```python
from build123d import *

# Parameters (mm, degrees)
MAIN_PLATE_DEPTH                 = 3
TOP_PLATE_CONNECTOR_HOLES_DEPTH  = 37.224942593
ZIPTIE_STRUCTURE_DEPTH           = 6
SKETCH5_W                        = 7.5
SKETCH5_H                        = 3
ZIPTIE_HOLES_DEPTH               = 52.45154631
REMOVING_STRESS_CONCENTRATIONS_R = 1.5


with BuildPart() as part:
    # Sketch1 → Main Plate (new body)
    with BuildSketch(Plane(origin=(0, 0, 0), x_dir=(1, 0, 0), z_dir=(0, 1, 0))):
        Polygon((-7, 25.526911935), (7, 25.526911935), (25.526911935, 7), (25.526911935, -7), (7, -25.526911935), (-7, -25.526911935), (-25.526911935, -7), (-25.526911935, 7), align=None)
    extrude(amount=MAIN_PLATE_DEPTH)

    # Sketch2 → Top Plate Connector Holes (cut, through all)
    with BuildSketch(Plane.XZ):
        Polygon((10.960155108, 18.03122292), (18.03122292, 10.960155108), (15.909902577, 8.838834765), (8.838834765, 15.909902577), align=None)
        Polygon((8.838834765, -15.909902577), (15.909902577, -8.838834765), (18.03122292, -10.960155108), (10.960155108, -18.03122292), align=None)
        Polygon((-15.909902577, -8.838834765), (-8.838834765, -15.909902577), (-10.960155108, -18.03122292), (-18.03122292, -10.960155108), align=None)
        Polygon((-8.838834765, 15.909902577), (-15.909902577, 8.838834765), (-18.03122292, 10.960155108), (-10.960155108, 18.03122292), align=None)
    extrude(amount=-TOP_PLATE_CONNECTOR_HOLES_DEPTH, mode=Mode.SUBTRACT)

    # Sketch3 → ZipTie Structure (add)
    with BuildSketch(Plane.XZ):
        Polygon((1.767766953, 19.445436483), (19.445436483, 1.767766953), (17.324116139, -0.353553391), (-0.353553391, 17.324116139), align=None)
        Polygon((-1.767766953, -19.445436483), (0.353553391, -17.324116139), (-17.324116139, 0.353553391), (-19.445436483, -1.767766953), align=None)
    extrude(amount=ZIPTIE_STRUCTURE_DEPTH)

    # Sketch5 → ZipTie Holes (cut, through all)
    with BuildSketch(Plane(origin=(-10.606601718, 0, -10.606601718), x_dir=(-0.7071067811865475, 0, 0.7071067811865477), z_dir=(-0.7071067811865477, 0, -0.7071067811865475))):
        with Locations((-5.75, -1.5)):
            Rectangle(SKETCH5_W, SKETCH5_H)
        with Locations((5.75, -1.5)):
            Rectangle(SKETCH5_W, SKETCH5_H)
    extrude(amount=-ZIPTIE_HOLES_DEPTH, mode=Mode.SUBTRACT)

    # Removing Stress Concentrations
    removing_stress_concentrations_edges = [part.edges().sort_by_distance(p)[0] for p in [
        (8.131727984, -3, 10.960155108),
        (10.960155108, -3, 8.131727984),
        (16.263455967, -3, 2.828427125),
        (-2.828427125, -3, -16.263455967),
        (-8.131727984, -3, -10.960155108),
        (-10.960155108, -3, -8.131727984),
        (-16.263455967, -3, -2.828427125),
        (2.828427125, -3, 16.263455967),
        (-16.263455967, 0, -2.828427125),
        (-8.131727984, 0, -10.960155108),
        (-0.707106781, 0, -18.384776311),
        (2.828427125, 0, 18.384776311),
        (10.606601718, 0, 10.606601718),
        (18.384776311, 0, 2.828427125),
        (10.960155108, 0, 8.131727984),
        (2.828427125, 0, 16.263455967),
        (0.707106781, -6, 18.384776311),
        (18.384776311, -6, 0.707106781),
        (18.384776311, 0, 0.707106781),
        (16.263455967, 0, 2.828427125),
        (0.707106781, 0, 18.384776311),
        (8.131727984, 0, 10.960155108),
        (-18.384776311, 0, -0.707106781),
        (-2.828427125, 0, -16.263455967),
        (-10.960155108, 0, -8.131727984),
        (-2.828427125, 0, -18.384776311),
        (-10.606601718, 0, -10.606601718),
        (-18.384776311, 0, -2.828427125),
        (-18.384776311, -6, -0.707106781),
        (-0.707106781, -6, -18.384776311),
    ]]
    fillet(removing_stress_concentrations_edges, radius=REMOVING_STRESS_CONCENTRATIONS_R - 0.0001)  # a hair under: the kernel refuses the full size


solid = part.part
```
Here's how the part is built. I have some questions about the finished solid (model axes, mm). A direction names the side the tool comes from. Give positions to 0.01 mm unless a question says otherwise; leave off trailing zeros. Write each loop counter-clockwise with the first axis right and the second up, starting at its lowest first coordinate (ties: lowest second). Pieces come first, ordered by that corner, then holes.
(1) Imagine slicing it at A-A, the plane y = -3.75. Write out the boundary of the cut face in (x, z), and give its area (3 significant figures).
Output values:
outline: (-19.45, -1.77) - (-1.77, -19.45) - (0.35, -17.32) - (-17.32, 0.35) - close; (-0.35, 17.32) - (17.32, -0.35) - (19.45, 1.77) - (1.77, 19.45) - close
area: 150 mm2
(2) On a 3-axis mill with a long thin cutter (end or side, diameter ignored), from which of +Z, -Z, +X, -X, +Y, -Y can I reach the whole of each face in a straight line? I mean faces 4 (the face through (18.858, -0.428, 0.543)), 5 (the face through (8.012, -0.428, 11.478)), 6 (the face through (-12.424, 1.479, -12.325)), 7 (the face through (-16.1, -0.43, -3.3)). Say none if no direction works.
Output values:
face 4: -Z, +X, -Y
face 5: +Z, -X
face 6: +Y, -Y
face 7: -Z, +X
(3) Will these pins go through, and if not, where does the flat tip stop? pin 1 (2 mm diameter, centred on x = 12, y = 1.5, fed in from +Z); pin 2 (4 mm diameter, centred on y = 1.5, z = -20.5, fed in from +X); pin 3 (1.5 mm diameter, centred on x = -16, z = 1, fed in from -Y); pin 4 (1 mm diameter, centred on x = -16.5, z = -17, fed in from -Y).
Output values:
pin 1: stops at z = 21.53
pin 2: stops at x = 14.03
pin 3: stops at y = 0
pin 4: passes through
(4) Imagine slicing it at B-B, the plane y = 1.25. Write out the boundary of the cut face in (x, z), and give its area (3 significant figures).
Output values:
outline: (-25.53, -7) - (-7, -25.53) - (7, -25.53) - (25.53, -7) - (25.53, 7) - (7, 25.53) - (-7, 25.53) - (-25.53, 7) - close; hole (-18.03, -10.96) - (-10.96, -18.03) - (-8.84, -15.91) - (-15.91, -8.84) - close; hole (-18.03, 10.96) - (-15.91, 8.84) - (-8.84, 15.91) - (-10.96, 18.03) - close; hole (8.84, -15.91) - (10.96, -18.03) - (18.03, -10.96) - (15.91, -8.84) - close; hole (8.84, 15.91) - (15.91, 8.84) - (18.03, 10.96) - (10.96, 18.03) - close
area: 1,800 mm2
(5) Thinking about a two-plate mould opening in X: for faces 1 (the face through (16.956, 1.479, -9.885)), 2 (the face through (25.527, 1, 0)), 3 (the face through (0.59, -0.43, 18.9)), which applies, pulls with the +X half, pulls with the -X half, needs draft (parallel to the pull), parting line crosses it, or undercut?
Output values:
face 1: undercut
face 2: pulls with the +X half
face 3: pulls with the -X half
(6) If I drill on L1, parallel to Z at x = 13, y = 1.5; L2, parallel to Z at x = 15, y = 0.5; L3, parallel to Y at x = 3.5, z = -7, over which ranges is the centre line in solid material (lowest first)?
Output values:
L1: z = -19.53 to -15.99, -11.75 to 11.75, 15.99 to 19.53
L2: z = -17.53 to -13.99, -9.75 to 9.75, 13.99 to 17.53
L3: y = 0 to 3
